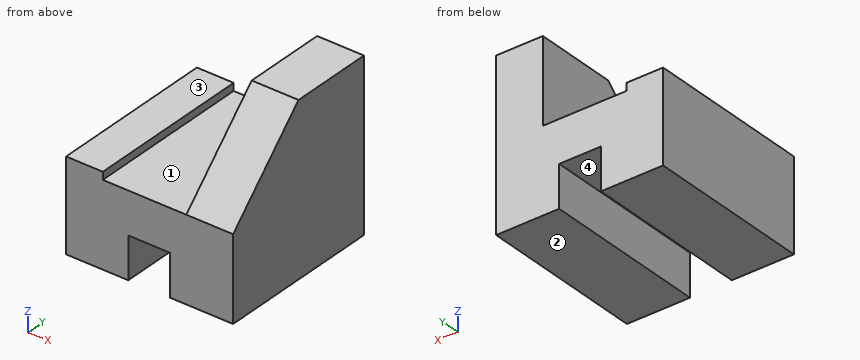
from build123d import *

# Parameters (mm, degrees)
F0_W     = 101.6
F0_H     = 101.6
F1_DEPTH = 101.6
F2_W     = 25.4
F2_H     = 25.4
F3_DEPTH = 232.918
F4_W     = 22.3325428724
F4_H     = 46.2064941585
F5_DEPTH = 115.824
F7_DEPTH = 154.94
F9_DEPTH = 54.356


with BuildPart() as f1:
    # F0 (on Top) → F1 (new body)
    with BuildSketch(Plane.XY):
        with Locations((-50.8, -50.8)):
            Rectangle(F0_W, F0_H)
    extrude(amount=F1_DEPTH)

    # F2 (on face) → F3 (cut)
    with BuildSketch(Plane.XZ.offset(101.6)):
        with Locations((-51.0816488743, 12.7)):
            Rectangle(F2_W, F2_H)
    extrude(amount=-F3_DEPTH, mode=Mode.SUBTRACT)

    # F4 (on face) → F5 (cut)
    with BuildSketch(Plane.XZ.offset(101.6)):
        with Locations((-90.4337285638, 78.4967529207)):
            Rectangle(F4_W, F4_H)
    extrude(amount=-F5_DEPTH, mode=Mode.SUBTRACT)

    # F6 (on face) → F7 (cut)
    with BuildSketch(Plane.XZ.offset(101.6)):
        Polygon((-28.4674571276, 101.6), (-79.2674571276, 101.6), (-79.2674571276, 55.3935058415), (-79.2674571276, 50.8), (-28.4674571276, 50.8), align=None)
    extrude(amount=-F7_DEPTH, mode=Mode.SUBTRACT)

    # F8 (on face) → F9 (cut)
    with BuildSketch(Plane.YZ):
        Polygon((-101.6, 101.6), (-101.6, 50.8), (-50.8, 101.6), align=None)
    extrude(amount=-F9_DEPTH, mode=Mode.SUBTRACT)


solid = f1.part
The model under review builds one solid part; all positions refer to its coordinate system, in mm. Face numbers are marked on the shaded views. A direction names the side the tool comes from. Round coordinates to 2 decimals unless told otherwise and drop trailing zeros. Loops run counter-clockwise (first coordinate to the right, second up) from the corner with the lowest first, then second, coordinate; pieces in that order, holes last. Notation, with made-up numbers: (46.25, 46.25) - (85.25, 46.25) arc R17 ccw to (85.25, 58.25) - close; hole circle Ø1 at (39, -19). An arc over 180 degrees is marked (long way). Use CSV: the item, a comma, the result in double quotes.
(1) Clearance check with flat-ended pins moving along their axes: P1, Ø6, axis at x = -43.5, y = -81.5, coming from the -Z side; P2, Ø11, axis at x = -89.5, y = -39.5, coming from the +Z side; P3, Ø4, axis at x = -57.5, y = -82.5, coming from the +Z side. State where each tip first meets the part, or that it passes through.
Working result:
P1,"stops at z = 25.4"
P2,"stops at z = 55.39"
P3,"stops at z = 50.8"
(2) Machinability: for the marked faces 1, 2, 3 and 4, which of the approach directions +Z, -Z, +X, -X, +Y, -Y give a long, thin tool a straight path to every point of the face, cutting with its end or side? Answer none if there is none.
Working result:
face 1,"+Z, +Y, -Y"
face 2,"-Z, +X, -X, +Y, -Y"
face 3,"+Z, -X, +Y, -Y"
face 4,"-Z, +Y, -Y"
(3) Take a section at A-A, the plane z = 7. Give the boundary of the cut face in (x, y), plus the area to 3 significant figures.
Working result:
outline,"(-101.6, -101.6) - (-63.78, -101.6) - (-63.78, 0) - (-101.6, 0) - close; (-38.38, -101.6) - (0, -101.6) - (0, 0) - (-38.38, 0) - close"
area,"7,740 mm^2"
(4) Take a section at D-D, the plane z = 53. Give the boundary of the cut face in (x, y).
Working result:
outline,"(-101.6, -101.6) - (-79.27, -101.6) - (-79.27, 0) - (-101.6, 0) - close; (-28.47, -99.4) - (0, -99.4) - (0, 0) - (-28.47, 0) - close"
(5) Take a section at B-B, the plane y = -63.5. Give the boundary of the cut face in (x, z), plus the area to 3 significant figures.
Working result:
outline,"(-101.6, 0) - (-63.78, 0) - (-63.78, 25.4) - (-38.38, 25.4) - (-38.38, 0) - (0, 0) - (0, 88.9) - (-28.47, 88.9) - (-28.47, 50.8) - (-79.27, 50.8) - (-79.27, 55.39) - (-101.6, 55.39) - close"
area,"5,700 mm^2"
(6) Take a section at C-C, the plane x = -24.5. Give the boundary of the cut face in (y, z).
Working result:
outline,"(-101.6, 0) - (0, 0) - (0, 101.6) - (-50.8, 101.6) - (-101.6, 50.8) - close"
(7) For line 1 (X direction, y = -8, z = 20); line 2 (X direction, y = -29, z = 52); line 3 (X direction, y = -12, z = 96), list the stretches that pass through material, from the lowest coordinate up.
Working result:
line 1,"x = -101.6 to -63.78, -38.38 to 0"
line 2,"x = -101.6 to -79.27, -28.47 to 0"
line 3,"x = -28.47 to 0"
